from build123d import *

# Parameters (mm, degrees)
SKETCH1_R      = 2.54
EXTRUDE1_DEPTH = 13.208
SKETCH2_R      = 3.175
EXTRUDE2_DEPTH = 0.6
EXTRUDE2_TAPER = 23
SKETCH3_R      = 3.175
EXTRUDE3_DEPTH = 0.6
EXTRUDE3_TAPER = 23


with BuildPart() as part:
    # Sketch1 → Extrude1 (new body)
    with BuildSketch(Plane.XY):
        with Locations((-108.082258725, 104.784469075)):
            Circle(SKETCH1_R)
    extrude(amount=-EXTRUDE1_DEPTH)

    # Sketch2 → Extrude2 (add)
    with BuildSketch(Plane.XY):
        with Locations((-108.082258725, 104.784469075)):
            Circle(SKETCH2_R)
    extrude(amount=EXTRUDE2_DEPTH, taper=EXTRUDE2_TAPER)

    # Sketch3 → Extrude3 (add)
    with BuildSketch(Plane(origin=(-216.039782036, 1.137132082, -13.208), x_dir=(-1, 0, 0), z_dir=(0, 0, -1))):
        with Locations((-107.957523311, 103.647336992)):
            Circle(SKETCH3_R)
    extrude(amount=EXTRUDE3_DEPTH, taper=EXTRUDE3_TAPER)


solid = part.part
For this review, take the finished solid that the model builds, in its own axes (mm). Give positions to 0.01 mm unless a question says otherwise; leave off trailing zeros. Loops run counter-clockwise (first coordinate to the right, second up) from the corner with the lowest first, then second, coordinate; pieces in that order, holes last. Notation, with made-up numbers: (46, 66) -> (60, 66) arc R16 cw to (60, 96) -> close; hole circle Ø9 at (84, 70.5). An arc over 180 degrees is marked (long way). One line per question, with ' | ' between items.
1) We need section A-A (z = -12.5). Write out the cut boundary in (x, y), plus the area to 3 significant figures.
Resolved:
outline: circle Ø5.08 at (-108.08, 104.78) | area: 20.3 mm2
2) The part is to be moulded in two halves that separate along Z. For faces 1 (the flat face through (-108, 105, -13.808)), 2 (the flat face through (-108, 105, 0.6)), 3 (the cylindrical face through (-105.736, 103.812, -6.512)), say which applies: +Z half, -Z half, draft (parallel to the pull), parting line (faces both ways), or undercut.
Resolved:
face 1: -Z half | face 2: +Z half | face 3: undercut
3) Insertion check: pin 1 Ø1.5 at (y, z) = (107, -4) entering from +X; pin 2 Ø3 at (y, z) = (105.5, -5) entering from +X; pin 3 Ø1.5 at (x, z) = (-109.5, -2) entering from -Y. Each pin has a flat end and moves straight along its axis. Give the tip position at first contact, or say it passes through.
Resolved:
pin 1: stops at x = -106.01 | pin 2: stops at x = -105.54 | pin 3: stops at y = 102.33
4) To check wall thickness, follow probe 1 along X at (y, z) = (104, -11.5); probe 2 along X at (y, z) = (103, -7); probe 3 along Y at (x, z) = (-107.75, -1.5). State the ranges of each line that lie inside material, in increasing order.
Resolved:
probe 1: x = -110.5 to -105.67 | probe 2: x = -109.89 to -106.27 | probe 3: y = 102.27 to 107.3
